Can you work these out from the model? Positions are in its coordinate system, mm. A direction names the side the tool comes from. Coordinates: 2 decimals unless noted, no trailing zeros. Write each loop counter-clockwise with the first axis right and the second up, starting at its lowest first coordinate (ties: lowest second). Pieces come first, ordered by that corner, then holes.
```python
from build123d import *

# Parameters (mm, degrees)
F0_W     = 211.1423015594
F0_H     = 71.8148499727
F1_DEPTH = 38.1
F4_DEPTH = 71.8148499727
F6_DEPTH = 90.678


with BuildPart() as f1:
    # F0 (on Top) → F1 (new body)
    with BuildSketch(Plane.XY):
        Rectangle(F0_W, F0_H)
    extrude(amount=F1_DEPTH)

    # F3 (on face) → F4 (join, through all)
    with BuildSketch(Plane.XZ.offset(35.9074249864)):
        Polygon((-8.89, 19.05), (8.89, 19.05), (8.89, 156.0654991746), (1.5875, 156.0654991746), (1.5875, 25.9591713548), (-1.5875, 25.9591713548), (-1.5875, 156.0654991746), (-8.89, 156.0654991746), align=None)
    extrude(amount=-F4_DEPTH)

    # F5 (on face) → F6 (cut)
    with BuildSketch(Plane.XZ.offset(35.9074249864)):
        with BuildLine():
            Line((-107.0431917906, 43.3599539101), (-107.0431917906, 3.6818189494))
            add(Edge.make_bspline(
                [(-107.0431917906, 3.6818189494), (-98.3908130965, 7.2554203267), (-78.2537077612, 18.3396192593), (-24.7400000825, 21.1928359311), (-8.89, 22.0728348941), (-8.89, 38.1)],
                knots=[0, 0, 0, 0, 0.3193478157, 0.7283198865, 1, 1, 1, 1], degree=3))
            Line((-8.89, 38.1), (-107.0431917906, 43.3599539101))
        make_face()
        with BuildLine():
            add(Edge.make_bspline(
                [(107.0431917906, 3.6818189494), (98.3908130965, 7.2554203267), (78.2537077612, 18.3396192593), (24.7400000825, 21.1928359311), (8.89, 22.0728348941), (8.89, 38.1)],
                knots=[0, 0, 0, 0, 0.3193478157, 0.7283198865, 1, 1, 1, 1], degree=3))
            Line((107.0431917906, 3.6818189494), (107.0431917906, 43.3599539101))
            Line((107.0431917906, 43.3599539101), (8.89, 38.1))
        make_face()
    extrude(amount=-F6_DEPTH, mode=Mode.SUBTRACT)


solid = f1.part
```
1. I'm going to push flat-ended pins straight in: P1, Ø1, axis at y = 22, z = 86, coming from the +X side; P2, Ø6, axis at y = 21.5, z = 120, coming from the -X side; P3, Ø10, axis at x = -22.5, y = -24, coming from the +Z side. Where does each tip first touch, or does it pass through?
2. If I drill on L1, parallel to X at y = 31, z = 52; L2, parallel to Z at x = 19.5, y = 6.5; L3, parallel to Z at x = 24, y = 21, over which ranges is the centre line in solid material (lowest first)?
3. We'd pull the mould along X, two halves only. Please class faces 1 (the face through (-5, -1, 156.065)), 2 (the face through (105.571, -1, 2)), 3 (the face through (-8.89, -1, 98)), 4 (the face through (1.588, -1, 98)): released by +X, released by -X, zero draft, split by the parting line, or undercut.
4. If we section it at A-A, the plane z = 104: List the corners of the cut face in (x, y) for me.
5. Which directions (+Z, -Z, +X, -X, +Y, -Y) give clear straight access to the entire face, cutting with the end or side of a thin tool? Please do faces 5 (the face through (-1.588, -1, 96)), 6 (the face through (-1, 1, 0)), 7 (the face through (8.89, -1, 96)).
Answers:
1. P1: stops at x = 8.89
1. P2: stops at x = -8.89
1. P3: stops at z = 21.97
2. L1: x = -8.89 to -1.59, 1.59 to 8.89
2. L2: z = 0 to 21.62
2. L3: z = 0 to 21.25
3. face 1: zero draft
3. face 2: released by +X
3. face 3: released by -X
3. face 4: undercut
4. outline: (-8.89, -35.91) - (-1.59, -35.91) - (-1.59, 35.91) - (-8.89, 35.91) - close; (1.59, -35.91) - (8.89, -35.91) - (8.89, 35.91) - (1.59, 35.91) - close
5. face 5: +Z, +Y, -Y
5. face 6: -Z, +X, -X, +Y, -Y
5. face 7: +Z, +X, +Y, -Y
